Can you work these out from the model? Positions are in its coordinate system, mm. A direction names the side the tool comes from. Round coordinates to 2 decimals unless told otherwise and drop trailing zeros. Order: outer loops, then holes, each group sorted by start corner. A loop starts at its lowest first (then second) coordinate and runs counter-clockwise, first axis right, second up.
Q1. If we section it at A-A (z = 30): Please give me the cut outline in (x, y), plus the area to 3 significant figures.
Q2. If we section it at B-B (z = -39): Please give me the cut outline in (x, y), plus the area to 3 significant figures.
Q3. If I drill on line 1 (Z direction, x = -9, y = 6); line 2 (Z direction, x = -22, y = 9.5); line 3 (Z direction, x = -50, y = 3), over which ranges is the centre line in solid material (lowest first)?
Q4. For faces 1 (the face through (-15, 6, -34.5)), 2 (the face through (-47.6, 8, -41.4)), 3 (the face through (-7.098, 6.631, -15.997)), 4 (the face through (-101, 6, -50)), which set-ups out of +Z, -Z, +X, -X, +Y, -Y let a thin tool reach every point of the face, with its end or its side?
Q5. We'd pull the mould along X, two halves only. Please class faces 5 (the face through (-15, 6, 34.5)), 6 (the face through (-55.495, 3.944, 39.242)), 7 (the face through (-15.043, 6.016, 18.364)), 8 (the face through (-200, 6, 1)): pulls with the +X half, pulls with the -X half, needs draft (parallel to the pull), parting line crosses it, or undercut.
Q6. Will these pins go through, and if not, where does the flat tip stop? P1, Ø9.5, axis at x = -150, z = -39, coming from the -Y side; P2, Ø3.5, axis at y = 6, z = 18, coming from the +X side.
from build123d import *

# Parameters (mm, degrees)
SKETCH1_W                                       = 200
SKETCH1_H                                       = 100
BOSS_EXTRUDE1_DEPTH                             = 12
CUT_EXTRUDE1_DEPTH                              = 207.504237245
CBORE_FOR_M5_SOCKET_HEAD_CAP_SCREW1_D           = 6
CBORE_FOR_M5_SOCKET_HEAD_CAP_SCREW1_CBORE_D     = 11
CBORE_FOR_M5_SOCKET_HEAD_CAP_SCREW1_CBORE_DEPTH = 8
M5X0_8_TAPPED_HOLE1_D                           = 4.2
M5X0_8_TAPPED_HOLE1_DEPTH                       = 14
M5X0_8_TAPPED_HOLE1_TIP                         = 1.2618073


with BuildPart() as part:
    # Sketch1 → Boss-Extrude1 (new body)
    with BuildSketch(Plane(origin=(0, 0, 0), x_dir=(1, 0, 0), z_dir=(0, 1, 0))):
        with Locations((-100, 0)):
            Rectangle(SKETCH1_W, SKETCH1_H)
    extrude(amount=BOSS_EXTRUDE1_DEPTH)

    # Sketch2 → Cut-Extrude1 (cut, through all)
    with BuildSketch(Plane(origin=(0, 12, 0), x_dir=(1, 0, 0), z_dir=(0, 1, 0))):
        with BuildLine():
            Line((-192, -25.5), (-178, -25.5))
            ThreePointArc((-178, -25.5), (-173.5, -30), (-178, -34.5))
            Line((-178, -34.5), (-192, -34.5))
            ThreePointArc((-192, -34.5), (-196.5, -30), (-192, -25.5))
        make_face()
        with BuildLine():
            Line((-192, 34.5), (-178, 34.5))
            ThreePointArc((-178, 34.5), (-173.5, 30), (-178, 25.5))
            Line((-178, 25.5), (-192, 25.5))
            ThreePointArc((-192, 25.5), (-196.5, 30), (-192, 34.5))
        make_face()
        with BuildLine():
            Line((-22, 34.5), (-8, 34.5))
            ThreePointArc((-8, 34.5), (-3.5, 30), (-8, 25.5))
            Line((-8, 25.5), (-22, 25.5))
            ThreePointArc((-22, 25.5), (-26.5, 30), (-22, 34.5))
        make_face()
        with BuildLine():
            Line((-22, -25.5), (-8, -25.5))
            ThreePointArc((-8, -25.5), (-3.5, -30), (-8, -34.5))
            Line((-8, -34.5), (-22, -34.5))
            ThreePointArc((-22, -34.5), (-26.5, -30), (-22, -25.5))
        make_face()
    extrude(amount=-CUT_EXTRUDE1_DEPTH, mode=Mode.SUBTRACT)

    # CBORE for M5 Socket Head Cap Screw1 (through all)
    with Locations(Plane.XZ):
        with Locations((-150, 39), (-50, 39), (-150, -39), (-50, -39)):
            CounterBoreHole(CBORE_FOR_M5_SOCKET_HEAD_CAP_SCREW1_D / 2, CBORE_FOR_M5_SOCKET_HEAD_CAP_SCREW1_CBORE_D / 2, CBORE_FOR_M5_SOCKET_HEAD_CAP_SCREW1_CBORE_DEPTH)

    # M5x0.8 Tapped Hole1
    with Locations(Plane(origin=(0, 0, 0), x_dir=(0, 0, -1), z_dir=(1, 0, 0))):
        with Locations((18, 6), (-18, 6)):
            Hole(M5X0_8_TAPPED_HOLE1_D / 2, depth=M5X0_8_TAPPED_HOLE1_DEPTH)
            with Locations((0, 0, -(M5X0_8_TAPPED_HOLE1_DEPTH + M5X0_8_TAPPED_HOLE1_TIP / 2))):  # 118° drill point
                Cone(0, M5X0_8_TAPPED_HOLE1_D / 2, M5X0_8_TAPPED_HOLE1_TIP, mode=Mode.SUBTRACT)


solid = part.part
Solution:
1. outline: (-200, 0) - (-196.5, 0) - (-196.5, 12) - (-200, 12) - close; (-173.5, 0) - (-26.5, 0) - (-26.5, 12) - (-173.5, 12) - close; (-3.5, 0) - (0, 0) - (0, 12) - (-3.5, 12) - close
1. area: 1,850 mm2
2. outline: (-200, 0) - (-155.5, 0) - (-155.5, 8) - (-153, 8) - (-153, 12) - (-200, 12) - close; (-147, 8) - (-144.5, 8) - (-144.5, 0) - (-55.5, 0) - (-55.5, 8) - (-53, 8) - (-53, 12) - (-147, 12) - close; (-47, 8) - (-44.5, 8) - (-44.5, 0) - (0, 0) - (0, 12) - (-47, 12) - close
2. area: 2,180 mm2
3. line 1: z = -50 to -34.5, -25.5 to -20.1, -15.9 to 15.9, 20.1 to 25.5, 34.5 to 50
3. line 2: z = -50 to -34.5, -25.5 to 25.5, 34.5 to 50
3. line 3: z = -50 to -44.5, -33.5 to 33.5, 44.5 to 50
4. face 1: +Y, -Y
4. face 2: -Y
4. face 3: +X
4. face 4: -Z, +X, -X, +Y, -Y
5. face 5: undercut
5. face 6: undercut
5. face 7: pulls with the +X half
5. face 8: pulls with the -X half
6. P1: stops at y = 8
6. P2: stops at x = -14.21
